from build123d import *

# Parameters (mm, degrees)
CYLINDER001_R           = 2
CYLINDER001_DEPTH       = 30
CYLINDER001_ROLL_ANGLE  = -90
CYLINDER002_R           = 11
CYLINDER002_DEPTH       = 7
CYLINDER002_PITCH_ANGLE = 90
CYLINDER003_R           = 10
CYLINDER003_DEPTH       = 10
CYLINDER003_PITCH_ANGLE = 90
PAD_DEPTH               = 10
BOX001_W                = 30
BOX001_H                = 10
BOX001_DEPTH            = 15
BOX002_W                = 10
BOX002_H                = 30
BOX002_DEPTH            = 40
BOX_W                   = 40
BOX_H                   = 30
BOX_DEPTH               = 10


with BuildPart() as cylinder001:
    # Cylinder001 → Cylinder001 (new body)
    with BuildSketch(Plane.XY):
        Circle(CYLINDER001_R)
    extrude(amount=CYLINDER001_DEPTH)


with BuildPart() as cylinder001_1:
    # Cylinder001 roll: moved
    add(cylinder001.part.rotate(Axis((0, 0, 0), (1, 0, 0)), CYLINDER001_ROLL_ANGLE))


with BuildPart() as cylinder001_2:
    # Cylinder001 placement: moved
    add(cylinder001_1.part.moved(Location((-15, -15, -15))))


with BuildPart() as bearing_cylinder:
    # Cylinder002 → Cylinder002 (new body)
    with BuildSketch(Plane.XY):
        Circle(CYLINDER002_R)
    extrude(amount=CYLINDER002_DEPTH)


with BuildPart() as bearing_cylinder_1:
    # Cylinder002 pitch: moved
    add(bearing_cylinder.part.rotate(Axis((0, 0, 0), (0, 1, 0)), CYLINDER002_PITCH_ANGLE))


with BuildPart() as bearing_cylinder_2:
    # Cylinder002 placement: moved
    add(bearing_cylinder_1.part.moved(Location((-18.5, 0, 0))))


with BuildPart() as bearing_cylinder_outer:
    # Cylinder003 → Cylinder003 (new body)
    with BuildSketch(Plane.XY):
        Circle(CYLINDER003_R)
    extrude(amount=CYLINDER003_DEPTH)


with BuildPart() as bearing_cylinder_outer_1:
    # Cylinder003 pitch: moved
    add(bearing_cylinder_outer.part.rotate(Axis((0, 0, 0), (0, 1, 0)), CYLINDER003_PITCH_ANGLE))


with BuildPart() as bearing_cylinder_outer_2:
    # Cylinder003 placement: moved
    add(bearing_cylinder_outer_1.part.moved(Location((-20, 0, 0))))


with BuildPart() as body:
    # Sketch → Pad (new body)
    with BuildSketch(Plane.XY):
        Polygon((6.928203, 0), (3.464102, 6), (-3.464102, 6), (-6.928203, 0), (-3.464102, -6), (3.464102, -6), align=None)
    extrude(amount=PAD_DEPTH)


with BuildPart() as body_1:
    # Body placement: moved
    add(body.part.moved(Location((10, 0, -20))))


with BuildPart() as negative_fusion:
    # Box001 → Box001 (new body)
    with BuildSketch(Plane(origin=(-20, -5, -20), x_dir=(1, 0, 0), z_dir=(0, 0, 1))):
        with Locations((15, 5)):
            Rectangle(BOX001_W, BOX001_H)
    extrude(amount=BOX001_DEPTH)

    # Fusion: union Cylinder001, Bearing Cylinder, Bearing Cylinder Outer, Body
    add(cylinder001_2.part)
    add(bearing_cylinder_2.part)
    add(bearing_cylinder_outer_2.part)
    add(body_1.part)


with BuildPart() as cube002:
    # Box002 → Box002 (new body)
    with BuildSketch(Plane(origin=(-20, -15, -20), x_dir=(1, 0, 0), z_dir=(0, 0, 1))):
        with Locations((5, 15)):
            Rectangle(BOX002_W, BOX002_H)
    extrude(amount=BOX002_DEPTH)


with BuildPart() as cut:
    # Box → Box (new body)
    with BuildSketch(Plane(origin=(-20, -15, -20), x_dir=(1, 0, 0), z_dir=(0, 0, 1))):
        with Locations((20, 15)):
            Rectangle(BOX_W, BOX_H)
    extrude(amount=BOX_DEPTH)

    # Fusion001: union Cube002
    add(cube002.part)

    # Cut: cut Negative Fusion
    add(negative_fusion.part, mode=Mode.SUBTRACT)


solid = cut.part
For this review, take the finished solid that the model builds, in its own axes (mm). A direction names the side the tool comes from. Give positions to 0.01 mm unless a question says otherwise; leave off trailing zeros. Order: outer loops, then holes, each group sorted by start corner. A loop starts at its lowest first (then second) coordinate and runs counter-clockwise, first axis right, second up. Notation, with made-up numbers: M -10.75,-2.5 L 43.25,-2.5 A33 ccw 43.25,32.5 Z; hole C -35.5,-9.5 d11. An arc over 180 degrees is marked long. Answer in a Markdown table with one row per item. Add a question column.
(1) For pin 1 (6 mm diameter, centred on y = 2, z = 5.5, fed in from +X); pin 2 (1.5 mm diameter, centred on x = 10, y = -7.5, fed in from +Z), all flat-tipped, find the tip position at first contact; note any pin that passes through.
(2) Consider section D-D on z = 6. State the section outline as (x, y) points.
(3) Consider section C-C on x = 2.5. State the section outline as (y, z) points, and give its area (3 significant figures).
(4) Consider section B-B on x = -15. State the section outline as (y, z) points.
(5) Mouldability with a two-part tool opening along X and no side actions: class faces 1 (the face through (10, 6, -15)), 2 (the face through (-15, 0, 11)), 3 (the face through (-10, 0, 11)), 4 (the face through (-19, 0, 10)) as +X half, -X half, draft (parallel to the pull), parting line (faces both ways), or undercut.
(6) Consider section A-A on z = -15. State the section outline as (x, y) points, and give its area (3 significant figures).
(7) Wall thickness on probe 1 along Y at (x, z) = (-16.5, 0); probe 2 along Y at (x, z) = (-17.5, 7.5); probe 3 along Z at (x, y) = (-10.7, 0): over which ranges is each line inside the solid? List them lowest first. Write a range as [from, to].
(8) For faces 5 (the face through (-18.5, 2, 10)), 6 (the face through (-7, -5, -14)), 7 (the face through (-11, 0, 10)), 8 (the face through (10, -6, -15)), list the 3-axis set-ups (+Z, -Z, +X, -X, +Y, -Y) from which the entire face can be reached by the end or side of a thin tool; tool diameter is ignored.
Evaluation:
| question | item | result |
|---|---|---|
| 1 | pin 1 | passes through |
| 1 | pin 2 | stops at z = -10 |
| 2 | outline | M -20,-15 L -10,-15 L -10,-8 L -11.5,-8 L -11.5,-9.22 L -18.5,-9.22 L -18.5,-8 L -20,-8 Z; M -20,8 L -18.5,8 L -18.5,9.22 L -11.5,9.22 L -11.5,8 L -10,8 L -10,15 L -20,15 Z |
| 3 | outline | M -15,-20 L -5,-20 L -5,-10 L -15,-10 Z; M 5,-20 L 15,-20 L 15,-10 L 5,-10 Z |
| 3 | area | 200 mm^2 |
| 4 | outline | M -15,-20 L -5,-20 L -5,-17 L -15,-17 Z; M -15,-13 L -5,-13 L -5,-9.8 A11 cw long 5,-9.8 L 5,-13 L 15,-13 L 15,20 L -15,20 Z; M 5,-20 L 15,-20 L 15,-17 L 5,-17 Z |
| 5 | face 1 | undercut |
| 5 | face 2 | undercut |
| 5 | face 3 | +X half |
| 5 | face 4 | draft |
| 6 | outline | M -20,-15 L -17,-15 L -17,-5 L -20,-5 Z; M -20,5 L -17,5 L -17,15 L -20,15 Z; M -13,-15 L 20,-15 L 20,15 L -13,15 L -13,5 L 5.96,5 L 6.54,6 L 13.46,6 L 16.93,0 L 13.46,-6 L 6.54,-6 L 5.96,-5 L -13,-5 Z |
| 6 | area | 750 mm^2 |
| 7 | probe 1 | y = [-15, -11], [11, 15] |
| 7 | probe 2 | y = [-15, -8.05], [8.05, 15] |
| 7 | probe 3 | z = [10, 20] |
| 8 | face 5 | none |
| 8 | face 6 | -Z, -X |
| 8 | face 7 | +X, -X |
| 8 | face 8 | +Z, -Z |
